```python
from build123d import *

# Parameters (mm, degrees)
BOSS_EXTRUDE1_DEPTH = 3.175
CUT_EXTRUDE1_DEPTH  = 7.35
CUT_EXTRUDE2_DEPTH  = 3.175
BOSS_EXTRUDE2_DEPTH = 3.175
SKETCH6_R           = 14.2875
CUT_EXTRUDE3_DEPTH  = 7.35
BOSS_EXTRUDE3_DEPTH = 6.35
SKETCH8_R           = 2.54
CUT_EXTRUDE4_DEPTH  = 7.35
SKETCH9_R           = 3.175
CUT_EXTRUDE5_DEPTH  = 7.35
FILLET1_R           = 25.4
FILLET2_R           = 9.525
FILLET4_R           = 6.35
FILLET3_R           = 50.8
SKETCH10_R          = 3.175
BOSS_EXTRUDE4_DEPTH = 6.35


with BuildPart() as part:
    # Sketch1 → Boss-Extrude1 (new body, symmetric)
    with BuildSketch(Plane(origin=(0, 0, 0), x_dir=(1, 0, 0), z_dir=(0, 1, 0))):
        with BuildLine():
            Line((76.2, 0), (173.0375, 0))
            ThreePointArc((173.0375, 0), (0, -173.0375), (-173.0375, 0))
            Line((-173.0375, 0), (-76.2, 0))
            ThreePointArc((-76.2, 0), (0, 76.2), (76.2, 0))
        make_face()
    extrude(amount=BOSS_EXTRUDE1_DEPTH, both=True)

    # Sketch2 → Cut-Extrude1 (cut, through all)
    with BuildSketch(Plane(origin=(0, 3.175, 0), x_dir=(1, 0, 0), z_dir=(0, 1, 0))):
        with BuildLine():
            Line((-78.965828786, -53.263124056), (-47.379497272, -31.957874433))
            ThreePointArc((-47.379497272, -31.957874433), (-52.988557288, -21.408766814), (-56.281763085, -9.923993354))
            Line((-56.281763085, -9.923993354), (-93.802938474, -16.539988923))
            ThreePointArc((-93.802938474, -16.539988923), (-88.314262147, -35.681278023), (-78.965828786, -53.263124056))
        make_face()
        with BuildLine():
            Line((-60.063484672, -148.662341282), (-45.196285496, -111.864732053))
            ThreePointArc((-45.196285496, -111.864732053), (-67.466623804, -100.023383129), (-86.788346911, -83.810532396))
            Line((-86.788346911, -83.810532396), (-115.337145237, -111.379786473))
            ThreePointArc((-115.337145237, -111.379786473), (-89.65959216, -132.92581179), (-60.063484672, -148.662341282))
        make_face()
        with BuildLine():
            Line((-35.681278023, -88.314262147), (-21.408766814, -52.988557288))
            ThreePointArc((-21.408766814, -52.988557288), (-31.957874433, -47.379497272), (-41.110269589, -39.699725872))
            Line((-41.110269589, -39.699725872), (-68.517115982, -66.166209786))
            ThreePointArc((-68.517115982, -66.166209786), (-53.263124056, -78.965828786), (-35.681278023, -88.314262147))
        make_face()
        with BuildLine():
            Line((-132.92581179, -89.65959216), (-100.023383129, -67.466623804))
            ThreePointArc((-100.023383129, -67.466623804), (-111.864732053, -45.196285496), (-118.817055401, -20.950652636))
            Line((-118.817055401, -20.950652636), (-157.901613099, -27.842314687))
            ThreePointArc((-157.901613099, -27.842314687), (-148.662341282, -60.063484672), (-132.92581179, -89.65959216))
        make_face()
        with BuildLine():
            Line((33.336040726, -156.833740933), (25.084545497, -118.013508029))
            ThreePointArc((25.084545497, -118.013508029), (0, -120.65), (-25.084545497, -118.013508029))
            Line((-25.084545497, -118.013508029), (-33.336040726, -156.833740933))
            ThreePointArc((-33.336040726, -156.833740933), (0, -160.3375), (33.336040726, -156.833740933))
        make_face()
        with BuildLine():
            Line((19.80358855, -93.16855897), (11.88215313, -55.901135382))
            ThreePointArc((11.88215313, -55.901135382), (0, -57.15), (-11.88215313, -55.901135382))
            Line((-11.88215313, -55.901135382), (-19.80358855, -93.16855897))
            ThreePointArc((-19.80358855, -93.16855897), (0, -95.25), (19.80358855, -93.16855897))
        make_face()
        with BuildLine():
            Line((115.337145237, -111.379786473), (86.788346911, -83.810532396))
            ThreePointArc((86.788346911, -83.810532396), (67.466623804, -100.023383129), (45.196285496, -111.864732053))
            Line((45.196285496, -111.864732053), (60.063484672, -148.662341282))
            ThreePointArc((60.063484672, -148.662341282), (89.65959216, -132.92581179), (115.337145237, -111.379786473))
        make_face()
        with BuildLine():
            Line((68.517115982, -66.166209786), (41.110269589, -39.699725872))
            ThreePointArc((41.110269589, -39.699725872), (31.957874433, -47.379497272), (21.408766814, -52.988557288))
            Line((21.408766814, -52.988557288), (35.681278023, -88.314262147))
            ThreePointArc((35.681278023, -88.314262147), (53.263124056, -78.965828786), (68.517115982, -66.166209786))
        make_face()
        with BuildLine():
            Line((157.901613099, -27.842314687), (118.817055401, -20.950652636))
            ThreePointArc((118.817055401, -20.950652636), (111.864732053, -45.196285496), (100.023383129, -67.466623804))
            Line((100.023383129, -67.466623804), (132.92581179, -89.65959216))
            ThreePointArc((132.92581179, -89.65959216), (148.662341282, -60.063484672), (157.901613099, -27.842314687))
        make_face()
        with BuildLine():
            Line((93.802938474, -16.539988923), (56.281763085, -9.923993354))
            ThreePointArc((56.281763085, -9.923993354), (52.988557288, -21.408766814), (47.379497272, -31.957874433))
            Line((47.379497272, -31.957874433), (78.965828786, -53.263124056))
            ThreePointArc((78.965828786, -53.263124056), (88.314262147, -35.681278023), (93.802938474, -16.539988923))
        make_face()
    extrude(amount=-CUT_EXTRUDE1_DEPTH, mode=Mode.SUBTRACT)

    # Sketch5 → Cut-Extrude2 (cut)
    with BuildSketch(Plane(origin=(0, 3.175, 0), x_dir=(1, 0, 0), z_dir=(0, 1, 0))):
        with BuildLine():
            Line((169.8625, 0), (173.0375, 0))
            ThreePointArc((173.0375, 0), (0, -173.0375), (-173.0375, 0))
            Line((-173.0375, 0), (-169.8625, 0))
            ThreePointArc((-169.8625, 0), (0, -169.8625), (169.8625, 0))
        make_face()
    extrude(amount=-CUT_EXTRUDE2_DEPTH, mode=Mode.SUBTRACT)

    # Sketch4 → Boss-Extrude2 (add, symmetric)
    with BuildSketch(Plane(origin=(0, 0, 0), x_dir=(1, 0, 0), z_dir=(0, 1, 0))):
        with BuildLine():
            Line((173.0375, 0), (195.2625, 0))
            ThreePointArc((195.2625, 0), (0, -195.2625), (-195.2625, 0))
            Line((-195.2625, 0), (-173.0375, 0))
            ThreePointArc((-173.0375, 0), (0, -173.0375), (173.0375, 0))
        make_face()
    extrude(amount=BOSS_EXTRUDE2_DEPTH, both=True)

    # Sketch6 → Cut-Extrude3 (cut, through all)
    with BuildSketch(Plane(origin=(0, 3.175, 0), x_dir=(1, 0, 0), z_dir=(0, 1, 0))):
        Circle(SKETCH6_R)
    extrude(amount=-CUT_EXTRUDE3_DEPTH, mode=Mode.SUBTRACT)

    # Sketch7 → Boss-Extrude3 (add, through all)
    with BuildSketch(Plane(origin=(0, 3.175, 0), x_dir=(1, 0, 0), z_dir=(0, 1, 0))):
        Polygon((32.206866836, -192.588062026), (53.968732111, -217.988062026), (101.069671923, -198.95804708), (103.466206527, -165.596461355), align=None)
    extrude(amount=-BOSS_EXTRUDE3_DEPTH)

    # Sketch8 → Cut-Extrude4 (cut, through all)
    with BuildSketch(Plane(origin=(0, 3.175, 0), x_dir=(-1, 0, 0), z_dir=(0, 1, 0))):
        with Locations((-72.677869349, 193.782658122)):
            Circle(SKETCH8_R)
    extrude(amount=-CUT_EXTRUDE4_DEPTH, mode=Mode.SUBTRACT)

    # Sketch9 → Cut-Extrude5 (cut, through all)
    with BuildSketch(Plane(origin=(0, 3.175, 0), x_dir=(1, 0, 0), z_dir=(0, 1, 0))):
        with Locations((-182.389864028, -25.4)):
            Circle(SKETCH9_R)
        with Locations((-120.900398056, -138.903982124)):
            Circle(SKETCH9_R)
        with Locations((0, -184.15)):
            Circle(SKETCH9_R)
        with Locations((182.389864028, -25.4)):
            Circle(SKETCH9_R)
    extrude(amount=-CUT_EXTRUDE5_DEPTH, mode=Mode.SUBTRACT)

    # Fillet1
    fillet1_edges = [part.edges().sort_by_distance(p)[0] for p in [
        (53.968732111, 0, 217.988062026),
        (101.069671923, 0, 198.95804708),
    ]]
    fillet(fillet1_edges, radius=FILLET1_R)

    # Fillet2
    fillet2_edges = [part.edges().sort_by_distance(p)[0] for p in [
        (-35.681278023, 0, 88.314262147),
        (-68.517115982, 0, 66.166209786),
        (-41.110269589, 0, 39.699725872),
        (-21.408766814, 0, 52.988557288),
        (33.336040726, 0, 156.833740933),
        (-33.336040726, 0, 156.833740933),
        (-25.084545497, 0, 118.013508029),
        (25.084545497, 0, 118.013508029),
        (-132.92581179, 0, 89.65959216),
        (-157.901613099, 0, 27.842314687),
        (-118.817055401, 0, 20.950652636),
        (-100.023383129, 0, 67.466623804),
        (19.80358855, 0, 93.16855897),
        (-19.80358855, 0, 93.16855897),
        (-11.88215313, 0, 55.901135382),
        (11.88215313, 0, 55.901135382),
        (115.337145237, 0, 111.379786473),
        (60.063484672, 0, 148.662341282),
        (45.196285496, 0, 111.864732053),
        (86.788346911, 0, 83.810532396),
        (93.802938474, 0, 16.539988923),
        (78.965828786, 0, 53.263124056),
        (47.379497272, 0, 31.957874433),
        (56.281763085, 0, 9.923993354),
        (157.901613099, 0, 27.842314687),
        (132.92581179, 0, 89.65959216),
        (100.023383129, 0, 67.466623804),
        (118.817055401, 0, 20.950652636),
        (68.517115982, 0, 66.166209786),
        (35.681278023, 0, 88.314262147),
        (21.408766814, 0, 52.988557288),
        (41.110269589, 0, 39.699725872),
        (-78.965828786, 0, 53.263124056),
        (-93.802938474, 0, 16.539988923),
        (-56.281763085, 0, 9.923993354),
        (-47.379497272, 0, 31.957874433),
        (-60.063484672, 0, 148.662341282),
        (-115.337145237, 0, 111.379786473),
        (-86.788346911, 0, 83.810532396),
        (-45.196285496, 0, 111.864732053),
    ]]
    fillet(fillet2_edges, radius=FILLET2_R)

    # Fillet4
    fillet4_edges = [part.edges().sort_by_distance(p)[0] for p in [
        (-195.2625, 0, 0),
        (195.2625, 0, 0),
        (32.206866836, 0, 192.588062026),
        (103.466206527, 0, 165.596461355),
    ]]
    fillet(fillet4_edges, radius=FILLET4_R)

    # Fillet3
    fillet3_edges = [part.edges().sort_by_distance(p)[0] for p in [
        (-76.2, 0, 0),
        (76.2, 0, 0),
    ]]
    fillet(fillet3_edges, radius=FILLET3_R)

    # Sketch10 → Boss-Extrude4 (add, through all)
    with BuildSketch(Plane(origin=(0, 3.175, 0), x_dir=(1, 0, 0), z_dir=(0, 1, 0))):
        with BuildLine():
            ThreePointArc((41.142321921, 185.080577729), (43.382996969, 107.81939227), (67.928946778, 34.526774967))
            ThreePointArc((67.928946778, 34.526774967), (8.977730657, 75.669282752), (-57.964006259, 49.463258873))
            ThreePointArc((-57.964006259, 49.463258873), (-16.94944122, 114.977483636), (3.307678079, 189.569422271))
            ThreePointArc((3.307678079, 189.569422271), (24.469422271, 206.242321921), (41.142321921, 185.080577729))
        make_face()
        with Locations((22.225, 187.325)):
            Circle(SKETCH10_R, mode=Mode.SUBTRACT)
    extrude(amount=-BOSS_EXTRUDE4_DEPTH)


solid = part.part
```
Geometry: final body of the model. Coordinates: model frame, mm. A direction names the side the tool comes from. Give positions to 0.01 mm unless a question says otherwise; leave off trailing zeros. Loops run counter-clockwise (first coordinate to the right, second up) from the corner with the lowest first, then second, coordinate; pieces in that order, holes last. Notation, with made-up numbers: (-15, 69.5) - (33, 69.5) arc R23 cw to (33, 86.5) - close; hole circle Ø1 at (74.25, -8). An arc over 180 degrees is marked (long way). Answer as CSV lines item,"result". Start each with the question number.
(1) Section query A-A (z = -55). Output: boundary loops of the cut face in (x, y) (1 decimal), and give its area (3 significant figures).
(2) Mould query, pull axis X, two halves, no side actions, for faces 1 (the face through (-3.74, 1.61, 169.82)), 2 (the face through (14, 3.175, 177)), 3 (the face through (55.147, -0.044, 212.222)). Classes: +X half, -X half, draft (parallel to the pull), parting line (faces both ways), or undercut.
(3) Ray query, line 1 along Z through (x, y) = (-52, -2.25); line 2 along X through (y, z) = (-1.5, 35.5); line 3 along Z through (x, y) = (-45, 1.5). Return the intervals inside material, ascending. Write a range as [from, to].
(4) Pin query (flat end, axial travel): P1, Ø2, axis at x = -152, y = -1, coming from the -Z side; P2, Ø2, axis at x = -48.5, y = 0.5, coming from the +Z side; P3, Ø3, axis at y = 2, z = -46, coming from the +X side. Return the tip coordinate at first contact, or that it passes through.
(5) Reachability of faces 4 (the face through (170.59, 0.04, 95.01)), 5 (the face through (-3.805, 1.61, 172.996)), 6 (the face through (-116.325, 0.044, 78.462)) from +Z, -Z, +X, -X, +Y, -Y: full face, straight path, thin tool, end or side. Return the list, or none.
Worked answers:
1,outline,"(-53.4, -3.2) - (58.6, -3.2) - (58.6, 3.2) - (-53.4, 3.2) - close"
1,area,"711 mm^2"
2,face 1,"undercut"
2,face 2,"draft"
2,face 3,"parting line"
3,line 1,"z = [-56.71, 23.71], [34.12, 50.22], [79.8, 109], [128.7, 188.21]"
3,line 2,"x = [-192.01, -156.1], [-115.31, -88.39], [-53.07, 53.07], [88.39, 115.31], [156.1, 192.01]"
3,line 3,"z = [-65.94, 44.12], [83.94, 163.79], [167.08, 190.01]"
4,P1,"stops at z = 0"
4,P2,"stops at z = 189.4"
4,P3,"stops at x = 63.12"
5,face 4,"+Z, +X, +Y, -Y"
5,face 5,"+Y"
5,face 6,"+Y, -Y"
